Autodesk Inventor part; units mm, degrees
ref_plane "YZ Plane" through (0, 0, 0) normal (1, 0, 0) x (0, 1, 0)
ref_plane "XZ Plane" through (0, 0, 0) normal (0, 1, 0) x (-1, 0, 0)
ref_plane "XY Plane" through (0, 0, 0) normal (0, 0, 1) x (1, 0, 0)
sketch "Sketch1" plane through (0, 0, 0) normal (0, 1, 0) x (-1, 0, 0)
  line L0 (38.1, 0) -> (38.1, -38.1)
  line L1 (0, -38.1) -> (0, 0)
  line L2 (0, 0) -> (0, 11.811)
  line L3 (0, 11.811) -> (38.1, 11.811)
  line L4 (38.1, 11.811) -> (38.1, 0)
  line L5 (0, -38.1) -> (0, -49.911)
  line L6 (0, -49.911) -> (38.1, -49.911)
  line L7 (38.1, -49.911) -> (38.1, -38.1)
  line L8 (-8.382, -38.1) -> (-8.382, -58.293)
  line L9 (-8.382, -58.293) -> (46.482, -58.293)
  line L10 (46.482, -58.293) -> (46.482, -38.1)
  line L11 (46.482, -38.1) -> (46.482, 0)
  line L12 (46.482, 0) -> (46.482, 20.193)
  line L13 (46.482, 20.193) -> (-8.382, 20.193)
  line L14 (-8.382, 20.193) -> (-8.382, 0)
  line L15 (-8.382, 0) -> (-8.382, -38.1)
  dimension "d0" = 38.1
  dimension "d1" = 38.1
  dimension "d2" = 11.811
  dimension "d3" = 11.811
  dimension "d4" = 8.382
extrude "Extrusion1" add sketch "Sketch1" along normal blind 3.81 contours L0 L7 L6 L5 L1 L2 L3 L4 | L15 L14 L13 L12 L11 L10 L9 L8
sketch "Sketch2" plane through (0, 3.81, 0) normal (0, 1, 0) x (1, 0, 0)
  line L0 (0, 0) -> (-38.1, 0)
  line L1 (-38.1, 0) -> (-38.1, 38.1)
  line L2 (-38.1, 38.1) -> (0, 38.1)
  line L3 (0, 38.1) -> (0, 0)
  dimension "d7" = 38.1
  dimension "d8" = 38.1
extrude "Extrusion2" cut sketch "Sketch2" against normal blind 13.6525
properties part number "peltier felt" material "Acetal Resin, Black"
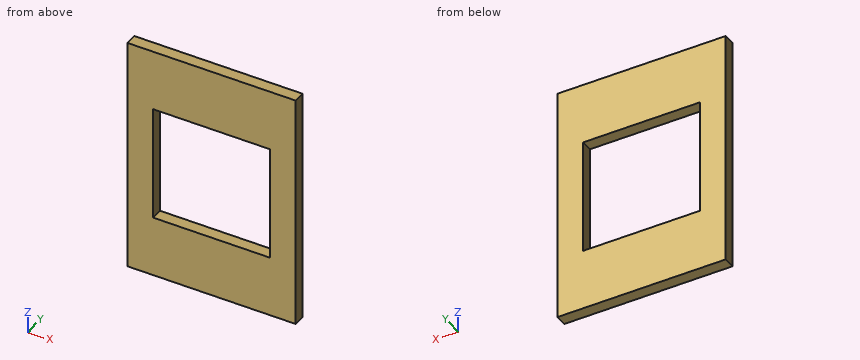
Check sheet for the modelled part. Datum: model origin and axes. Units: mm. Round coordinates to 2 decimals unless told otherwise and drop trailing zeros. Write each loop counter-clockwise with the first axis right and the second up, starting at its lowest first coordinate (ties: lowest second). Pieces come first, ordered by that corner, then holes. Notation, with made-up numbers: M 58.25,26 L 85.25,26 A17 ccw 85.25,59 Z; hole C 0,86.5 d3. An arc over 180 degrees is marked long. Write item = value, one per line. Start each with the question number.
1. Section check C-C, the plane y = 2.75. Record the cut outline in (x, z), then the cut area to 3 significant figures.
2. Gauge pin test, flat end, axial feed: pin 1 (1.5 mm diameter, centred on x = -0.5, z = -7.5, fed in from +Y). Record the tip position at first contact, or that the pin passes through.
3. Scan lines: line 1 (Z direction, x = -14.5, y = 0.4); line 2 (X direction, y = 0.75, z = -7). Record each from-to range of solid material in increasing order. Write a range as [from, to].
4. Section check A-A, the plane z = -33. Record the cut outline in (x, y), then the cut area to 3 significant figures.
5. Section check B-B, the plane x = -25.5. Record the cut outline in (y, z).
Results found:
q1.outline = M -46.48,-58.29 L 8.38,-58.29 L 8.38,20.19 L -46.48,20.19 Z; hole M -38.1,-38.1 L 0,-38.1 L 0,0 L -38.1,0 Z
q1.area = 2,850 mm^2
q2.pin_1 = 3.81
q3.line_1 = [-58.29, -38.1], [0, 20.19]
q3.line_2 = [-46.48, -38.1], [0, 8.38]
q4.outline = M -46.48,0 L -38.1,0 L -38.1,3.81 L -46.48,3.81 Z; M 0,0 L 8.38,0 L 8.38,3.81 L 0,3.81 Z
q4.area = 63.9 mm^2
q5.outline = M 0,-58.29 L 3.81,-58.29 L 3.81,-38.1 L 0,-38.1 Z; M 0,0 L 3.81,0 L 3.81,20.19 L 0,20.19 Z
